Work out the finished part from the listing and answer in its coordinate system (mm). Give positions to 0.01 mm unless a question says otherwise; leave off trailing zeros. Order: outer loops, then holes, each group sorted by start corner. A loop starts at its lowest first (then second) coordinate and runs counter-clockwise, first axis right, second up. Notation, with made-up numbers: (39, 77.25) - (43, 77.25) arc R31 cw to (43, 111.25) - close; hole circle Ø9 at (30, -1). An arc over 180 degrees is marked (long way). Write each question's results on one line, items separated by ' | '.
from build123d import *

# Parameters (mm, degrees)
SKETCH1_R               = 80
BOSS_EXTRUDE1_DEPTH     = 3
SKETCH2_W               = 3
SKETCH2_H               = 14
SKETCH2_W_2             = 14
SKETCH2_H_2             = 3
CUT_EXTRUDE1_DEPTH      = 3
CUT_EXTRUDE3_DEPTH      = 1
CUT_EXTRUDE3_DEPTH_BACK = 3
CUT_EXTRUDE4_DEPTH      = 1
CUT_EXTRUDE4_DEPTH_BACK = 3
CUT_EXTRUDE5_DEPTH      = 1
CUT_EXTRUDE5_DEPTH_BACK = 3
CUT_EXTRUDE6_DEPTH      = 1
CUT_EXTRUDE6_DEPTH_BACK = 3
SKETCH7_R               = 7
CUT_EXTRUDE7_DEPTH      = 3


with BuildPart() as part:
    # Sketch1 → Boss-Extrude1 (new body)
    with BuildSketch(Plane(origin=(0, 0, 0), x_dir=(1, 0, 0), z_dir=(0, 1, 0))):
        Circle(SKETCH1_R)
    extrude(amount=BOSS_EXTRUDE1_DEPTH)

    # Sketch2 → Cut-Extrude1 (cut)
    with BuildSketch(Plane(origin=(0, 3, 0), x_dir=(1, 0, 0), z_dir=(0, 1, 0))):
        with Locations((0, 20)):
            Rectangle(SKETCH2_W, SKETCH2_H)
        with Locations((0, 60)):
            Rectangle(SKETCH2_W, SKETCH2_H)
        with Locations((-20, 0)):
            Rectangle(SKETCH2_W_2, SKETCH2_H_2)
        with Locations((-60, 0)):
            Rectangle(SKETCH2_W_2, SKETCH2_H_2)
        with Locations((20, 0)):
            Rectangle(SKETCH2_W_2, SKETCH2_H_2)
        with Locations((60, 0)):
            Rectangle(SKETCH2_W_2, SKETCH2_H_2)
        with Locations((0, -20)):
            Rectangle(SKETCH2_W, SKETCH2_H)
        with Locations((0, -60)):
            Rectangle(SKETCH2_W, SKETCH2_H)
        with Locations((-15, -45)):
            Rectangle(SKETCH2_W_2, SKETCH2_H_2)
        with Locations((15, -45)):
            Rectangle(SKETCH2_W_2, SKETCH2_H_2)
        with Locations((-45, -45)):
            Rectangle(SKETCH2_W_2, SKETCH2_H_2)
        with Locations((45, -45)):
            Rectangle(SKETCH2_W_2, SKETCH2_H_2)
    extrude(amount=-CUT_EXTRUDE1_DEPTH, mode=Mode.SUBTRACT)

    # Sketch3 → Cut-Extrude3 (cut, two sides)
    with BuildSketch(Plane(origin=(0, 3, 0), x_dir=(1, 0, 0), z_dir=(0, 1, 0))) as cut_extrude3_sk:
        Polygon((-465.463683449, 40), (-69.282032303, 40), (-54, 40), (-54, 59.025418253), (-54, 455.2070694), (-616.816816127, 1012.949693112), (-1028.280499576, 597.742623712), align=None)
    extrude(amount=CUT_EXTRUDE3_DEPTH, mode=Mode.SUBTRACT)
    extrude(cut_extrude3_sk.sketch, amount=-CUT_EXTRUDE3_DEPTH_BACK, mode=Mode.SUBTRACT)

    # Sketch4 → Cut-Extrude4 (cut, two sides)
    with BuildSketch(Plane(origin=(0, 3, 0), x_dir=(1, 0, 0), z_dir=(0, 1, 0))) as cut_extrude4_sk:
        Polygon((465.463683449, 40), (69.282032303, 40), (54, 40), (54, 59.025418253), (54, 455.2070694), (616.816816127, 1012.949693112), (1028.280499576, 597.742623712), align=None)
    extrude(amount=CUT_EXTRUDE4_DEPTH, mode=Mode.SUBTRACT)
    extrude(cut_extrude4_sk.sketch, amount=-CUT_EXTRUDE4_DEPTH_BACK, mode=Mode.SUBTRACT)

    # Sketch5 → Cut-Extrude5 (cut, two sides)
    with BuildSketch(Plane(origin=(0, 3, 0), x_dir=(1, 0, 0), z_dir=(0, 1, 0))) as cut_extrude5_sk:
        Polygon((-431.335496535, 70), (-38.729833462, 70), (-9.5, 70), (-9.5, 79.433934814), (-9.5, 472.039597887), (-551.23098741, 1040.444703413), (-973.066483945, 638.405105526), align=None)
    extrude(amount=CUT_EXTRUDE5_DEPTH, mode=Mode.SUBTRACT)
    extrude(cut_extrude5_sk.sketch, amount=-CUT_EXTRUDE5_DEPTH_BACK, mode=Mode.SUBTRACT)

    # Sketch6 → Cut-Extrude6 (cut, two sides)
    with BuildSketch(Plane(origin=(0, 3, 0), x_dir=(1, 0, 0), z_dir=(0, 1, 0))) as cut_extrude6_sk:
        Polygon((431.335496535, 70), (38.729833462, 70), (9.5, 70), (9.5, 79.433934814), (9.5, 472.039597887), (551.23098741, 1040.444703413), (973.066483945, 638.405105526), align=None)
    extrude(amount=CUT_EXTRUDE6_DEPTH, mode=Mode.SUBTRACT)
    extrude(cut_extrude6_sk.sketch, amount=-CUT_EXTRUDE6_DEPTH_BACK, mode=Mode.SUBTRACT)

    # Sketch7 → Cut-Extrude7 (cut)
    with BuildSketch(Plane(origin=(0, 3, 0), x_dir=(1, 0, 0), z_dir=(0, 1, 0))):
        with Locations((-15, -23.5)):
            Circle(SKETCH7_R)
        with Locations((15, -23.5)):
            Circle(SKETCH7_R)
    extrude(amount=-CUT_EXTRUDE7_DEPTH, mode=Mode.SUBTRACT)


solid = part.part
1. Straight lines are drawn through the part: line 1 (Z direction, x = -15, y = 2.3); line 2 (X direction, y = 2.25, z = 23.5); line 3 (X direction, y = 2.65, z = 21.5). For each, find the intervals that lie inside material, in ascending order. Write a range as [from, to].
Answer list:
line 1: [-70, -1.5], [1.5, 16.5], [30.5, 43.5], [46.5, 78.58] | line 2: [-76.47, -22], [-8, -1.5], [1.5, 8], [22, 76.47] | line 3: [-77.06, -21.71], [-8.29, -1.5], [1.5, 8.29], [21.71, 77.06]
2. A cutting plane is placed at B-B, the plane x = 15. Write down the section's boundary in (y, z).
Answer list:
outline: (0, -70) - (3, -70) - (3, -1.5) - (0, -1.5) - close; (0, 1.5) - (3, 1.5) - (3, 16.5) - (0, 16.5) - close; (0, 30.5) - (3, 30.5) - (3, 43.5) - (0, 43.5) - close; (0, 46.5) - (3, 46.5) - (3, 78.58) - (0, 78.58) - close
3. Given P1, Ø1.5, axis at y = 2, z = -60, coming from the +X side; P2, Ø1.5, axis at y = 1, z = 45, coming from the -X side; P3, Ø0.9, axis at x = 20.5, y = 1, coming from the -Z side; P4, Ø12.5, axis at x = 15, z = 23.5, coming from the +Y side, each flat-ended and moving along its own axis, determine where each tip first touches the part or whether it passes through.
Answer list:
P1: x = 53.75 | P2: x = -66.65 | P3: z = -70 | P4: through
4. A cutting plane is placed at D-D, the plane x = 44. Write down the section's boundary in (y, z).
Answer list:
outline: (0, -66.81) - (3, -66.81) - (3, 43.5) - (0, 43.5) - close; (0, 46.5) - (3, 46.5) - (3, 66.81) - (0, 66.81) - close
5. A cutting plane is placed at C-C, the plane z = 63. Write down the section's boundary in (x, y), then the cut area to 3 significant figures.
Answer list:
outline: (-49.31, 0) - (-1.5, 0) - (-1.5, 3) - (-49.31, 3) - close; (1.5, 0) - (49.31, 0) - (49.31, 3) - (1.5, 3) - close | area: 287 mm^2
6. A cutting plane is placed at A-A, the plane z = 23.5. Write down the section's boundary in (x, y), then the cut area to 3 significant figures.
Answer list:
outline: (-76.47, 0) - (-22, 0) - (-22, 3) - (-76.47, 3) - close; (-8, 0) - (-1.5, 0) - (-1.5, 3) - (-8, 3) - close; (1.5, 0) - (8, 0) - (8, 3) - (1.5, 3) - close; (22, 0) - (76.47, 0) - (76.47, 3) - (22, 3) - close | area: 366 mm^2
7. Determine the mould class of faces 1 (the face through (-20.555, 1.521, 27.759)), 2 (the face through (-2.345, 1.479, 79.966)), 3 (the face through (46.796, 1.479, -64.886)), 4 (the face through (-1, 0, -1)) for opening direction Z: +Z half, -Z half, draft (parallel to the pull), parting line (faces both ways), or undercut.
Answer list:
face 1: undercut | face 2: parting line | face 3: -Z half | face 4: draft
